Solid Edge part; units mm, degrees
sketch "Sketch1" plane through (0, 0, 0) normal (0, 0, 1) x (1, 0, 0)
  circle A0 centre (0, 0) radius 10.16
  circle A1 centre (0, 0) radius 2.54
extrude "Protrusion1" add sketch "Sketch1" along normal blind 10.16
sketch "Sketch2" plane through (0, 0, 10.16) normal (0, 0, 1) x (1, 0, 0)
  circle A0 centre (0, 0) radius 6.35
extrude "ExtrudedProtrusion_3" add sketch "Sketch2" along normal blind 2.54
CAD build for the part. Positions are in the model's coordinates, mm. A direction names the side the tool comes from. Round coordinates to 2 decimals unless told otherwise and drop trailing zeros. Write each loop counter-clockwise with the first axis right and the second up, starting at its lowest first coordinate (ties: lowest second). Pieces come first, ordered by that corner, then holes. Notation, with made-up numbers: M 80,10.25 L 104,10.25 A28 ccw 104,41.25 Z; hole C 86,76.5 d11. An arc over 180 degrees is marked long. Use a Markdown table: item, result. Add a question column.
1. Flat gauge pins, fed straight in: P1, Ø2, axis at y = 0.5, z = 7.5, coming from the -X side; P2, Ø6, axis at x = 5, z = 4, coming from the -Y side; P3, Ø5, axis at x = 3, z = 11, coming from the +Y side; P4, Ø2, axis at y = -7.5, z = 9.5, coming from the +X side. Where does each tip first touch, or does it go through?
2. 3-axis set-ups, long thin cutter, end or side, ignore diameter. For faces 4 (the face through (-1.38, 6.2, 11.41)), 5 (the face through (0, 0, 12.7)), 6 (the face through (-0.33, -2.52, 5.01)): which of +Z, -Z, +X, -X, +Y, -Y reach the whole face in a straight line?
3. Pull direction Y, two halves, no side cores. Call faces 1 (the face through (0, 0, 10.16)), 2 (the face through (-1.323, -10.074, 5.009)), 3 (the face through (2, -2, 0)): released by +Y, released by -Y, zero draft, split by the parting line, or undercut.
4. Drill centre lines: probe 1 along Y at (x, z) = (0, 6); probe 2 along Z at (x, y) = (6.25, 6.5); probe 3 along Z at (x, y) = (0.75, 0.25). Where is each one in solid material? Low to high.
5. Slice it at D-D on z = 3.25. Give the cut face in (x, y).
6. Slice it at A-A on x = 0. Give the cut face in (y, z).
7. Slice it at C-C on z = 10.5. Give the cut face in (x, y), then the cut area to 3 significant figures.
Reply:
| question | item | result |
|---|---|---|
| 1 | P1 | stops at x = -10.16 |
| 1 | P2 | stops at y = -9.96 |
| 1 | P3 | stops at y = 10.14 |
| 1 | P4 | stops at x = 7.81 |
| 2 | face 4 | +Z |
| 2 | face 5 | +Z, +X, -X, +Y, -Y |
| 2 | face 6 | -Z |
| 3 | face 1 | undercut |
| 3 | face 2 | split by the parting line |
| 3 | face 3 | zero draft |
| 4 | probe 1 | y = -10.16 to -2.54, 2.54 to 10.16 |
| 4 | probe 2 | z = 0 to 10.16 |
| 4 | probe 3 | z = 10.16 to 12.7 |
| 5 | outline | C 0,0 d20.32; hole C 0,0 d5.08 |
| 6 | outline | M -10.16,0 L -2.54,0 L -2.54,10.16 L 2.54,10.16 L 2.54,0 L 10.16,0 L 10.16,10.16 L 6.35,10.16 L 6.35,12.7 L -6.35,12.7 L -6.35,10.16 L -10.16,10.16 Z |
| 7 | outline | C 0,0 d12.7 |
| 7 | area | 127 mm^2 |
